Here's how the part is built. I have some questions about the finished solid (model axes, mm). Give positions to 0.01 mm unless a question says otherwise; leave off trailing zeros. Write each loop counter-clockwise with the first axis right and the second up, starting at its lowest first coordinate (ties: lowest second). Pieces come first, ordered by that corner, then holes. Notation, with made-up numbers: (33.5, 31.5) -> (56.5, 31.5) arc R9 ccw to (56.5, 43.5) -> close; hole circle Ø6 at (79.25, -34). An arc over 180 degrees is marked (long way). Use one line per item in the form item = value.
```python
from build123d import *

# Parameters (mm, degrees)
F1_DEPTH = 12.7


with BuildPart() as f1:
    # F0 (on Top) → F1 (new body)
    with BuildSketch(Plane.XY):
        Polygon((-246.38, 152.4), (-292.1, 152.4), (-292.1, 127), (-304.8, 127), (-304.8, 101.6), (-292.1, 101.6), (-292.1, 76.2), (-304.8, 76.2), (-304.8, 50.8), (-292.1, 50.8), (-292.1, 25.4), (-304.8, 25.4), (-304.8, 0), (-292.1, 0), (-292.1, -25.4), (-304.8, -25.4), (-304.8, -50.8), (-292.1, -50.8), (-292.1, -76.2), (-304.8, -76.2), (-304.8, -101.6), (-292.1, -101.6), (-292.1, -127), (-304.8, -127), (-304.8, -152.4), (304.8, -152.4), (304.8, -127), (292.1, -127), (292.1, -101.6), (304.8, -101.6), (304.8, -76.2), (292.1, -76.2), (292.1, -50.8), (304.8, -50.8), (304.8, -25.4), (292.1, -25.4), (292.1, 0), (304.8, 0), (304.8, 25.4), (292.1, 25.4), (292.1, 50.8), (304.8, 50.8), (304.8, 76.2), (292.1, 76.2), (292.1, 101.6), (304.8, 101.6), (304.8, 127), (292.1, 127), (292.1, 152.4), (266.7, 152.4), (266.7, 139.7), (241.3, 139.7), (241.3, 152.4), (144.78, 152.4), (144.78, 139.7), (119.38, 139.7), (119.38, 152.4), (22.86, 152.4), (22.86, 139.7), (-2.54, 139.7), (-2.54, 152.4), (-99.06, 152.4), (-99.06, 139.7), (-124.46, 139.7), (-124.46, 152.4), (-220.98, 152.4), (-220.98, 139.7), (-246.38, 139.7), align=None)
    extrude(amount=F1_DEPTH)


solid = f1.part
```
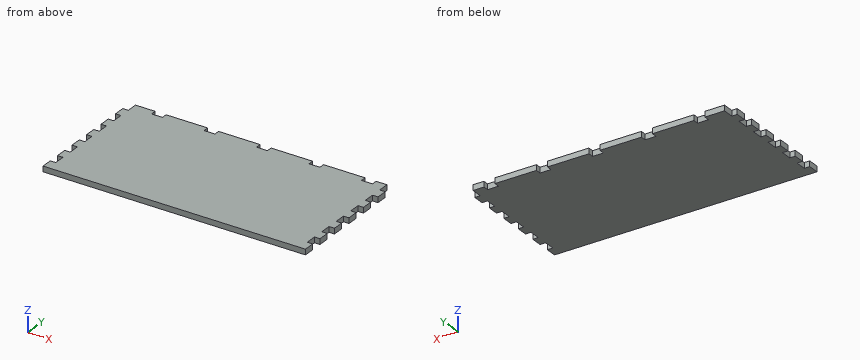
Q1. Will these pins go through, and if not, where does the flat tip stop? pin 1 Ø6.5 at (x, z) = (297, 6.5) entering from +Y; pin 2 Ø4 at (y, z) = (43.5, 4.5) entering from -X; pin 3 Ø4 at (x, z) = (134.5, 6.5) entering from +Y.
Result set:
pin_1 = 127
pin_2 = -292.1
pin_3 = 139.7
Q2. If I drill on line 1 along X through (y, z) = (140.5, 5.5); line 2 along X through (y, z) = (-23, 5.5); line 3 along Y through (x, z) = (127, 4), over which ranges is the centre line in solid material (lowest first)? Write a range as from..to.
Result set:
line_1 = -292.1..-246.38, -220.98..-124.46, -99.06..-2.54, 22.86..119.38, 144.78..241.3, 266.7..292.1
line_2 = -292.1..292.1
line_3 = -152.4..139.7
Q3. I want a section at A-A, the plane y = -58. Write out the boundary of the cut face in (x, z), and give its area (3 significant figures).
Result set:
outline = (-292.1, 0) -> (292.1, 0) -> (292.1, 12.7) -> (-292.1, 12.7) -> close
area = 7,420 mm2
